Autodesk Inventor part; units mm, degrees
ref_plane "YZ Plane" through (0, 0, 0) normal (1, 0, 0) x (0, 1, 0)
ref_plane "XZ Plane" through (0, 0, 0) normal (0, 1, 0) x (-1, 0, 0)
ref_plane "XY Plane" through (0, 0, 0) normal (0, 0, 1) x (1, 0, 0)
sketch "스케치1" plane through (0, 0, 0) normal (0, 1, 0) x (-1, 0, 0)
  circle A0 centre (0, 0) radius 3.4
  dimension "d0" = 6.8
extrude "돌출1" add sketch "스케치1" along normal blind 3.8
hole "구멍1" at (0, 3.8, 0) direction (0, -1, 0) diameter 2.5 end through all
hole "구멍2" at (0, 3.8, 0) direction (0, -1, 0) diameter 4.6 depth 1.1
hole "구멍3" at (0, 0, 0) direction (0, 1, 0) diameter 4.6 depth 2.1
sketch "스케치2" plane through (0, 3.8, 0) normal (0, 1, 0) x (1, 0, 0)
  line L0 (0, 3.4) -> (0, -16)
  line L1 (-2.6, -2.1909) -> (-1.2931, -14.8337)
  arc A0 (0, 3.4) -> (-2.6, -2.1909) centre (0, 0) ccw
  arc A1 (-1.2931, -14.8337) -> (0, -16) centre (0, -14.7) ccw
  line L2 (2.6, -2.1909) -> (1.2931, -14.8337)
  arc A2 (2.6, -2.1909) -> (0, 3.4) centre (0, 0) ccw
  arc A3 (0, -16) -> (1.2931, -14.8337) centre (0, -14.7) ccw
  arc A4 (-2.6, -2.1909) -> (2.6, -2.1909) centre (0, 0) ccw
  dimension "d34" = 19.4
extrude "돌출2" add sketch "스케치2" against normal blind 1.4 contours A4 L2 A3 L0 | L0 A1 L1 A4
properties part number "SG90 SingleArm"
Design review of the part built by this model. Coordinates are the model's own, in mm. A direction names the side the tool comes from. Give positions to 0.01 mm unless a question says otherwise; leave off trailing zeros. Write each loop counter-clockwise with the first axis right and the second up, starting at its lowest first coordinate (ties: lowest second). Pieces come first, ordered by that corner, then holes. Notation, with made-up numbers: (-6, -4) - (41, -4) arc R16 ccw to (41, 27) - close; hole circle Ø3 at (-12, -35). An arc over 180 degrees is marked (long way). Return JSON: item names as keys, results as strings. Group by question number.
(1) We need section C-C, the plane y = 1.9. Give the boundary of the cut face in (x, z), then the cut area to 3 significant figures.
(2) Mouldability with a two-part tool opening along X and no side actions: class faces 4 (the cylindrical face through (1.4, 3.242, -1.825)), 5 (the flat face through (0, 3.8, 6)), 6 (the flat face through (-2, 3, 8)) as +X half, -X half, draft (parallel to the pull), parting line (faces both ways), or undercut.
(3) We need section B-B, the plane x = 1. Give the boundary of the cut face in (y, z), then the cut area to 3 significant figures.
(4) Insertion check: pin 1 (1 mm diameter, centred on y = 2.5, z = 11, fed in from +X); pin 2 (2 mm diameter, centred on x = 1, z = 11, fed in from -Y); pin 3 (4 mm diameter, centred on x = 0, z = 0, fed in from +Y); pin 4 (2 mm diameter, centred on x = 0, z = 0, fed in from +Y). Each pin has a flat end and moves straight along its axis. Give the tip position at first contact, or say it passes through.
(5) We need section A-A, the plane z = 0. Give the boundary of the cut face in (x, y).
(6) To check wall thickness, follow probe 1 along Z at (x, y) = (0, 2.55); probe 2 along Z at (x, y) = (0, 3.2); probe 3 along Y at (x, z) = (1, 6.5). State the ranges of each line that lie inside material, in increasing order.
(7) We need section D-D, the plane x = -1.5. Give the boundary of the cut face in (y, z), then the cut area to 3 significant figures.
(8) Machinability: for faces 1 (the cylindrical face through (0.44, 1.87, -3.37)), 2 (the flat face through (1, 2.7, 1)), 3 (the flat face through (2, 3, 8)), which of the approach directions +Z, -Z, +X, -X, +Y, -Y give a long, thin tool a straight path to every point of the face, cutting with its end or side? Answer none if there is none.
Reported:
{
 "1": {"outline": "circle Ø6.8 at (0, 0); hole circle Ø4.6 at (0, 0)", "area": "19.7 mm2"},
 "2": {"face 4": "undercut", "face 5": "draft", "face 6": "-X half"},
 "3": {"outline": "(0, -3.25) - (3.8, -3.25) - (3.8, -2.07) - (2.7, -2.07) - (2.7, -0.75) - (2.1, -0.75) - (2.1, -2.07) - (0, -2.07) - close; (0, 2.07) - (2.1, 2.07) - (2.1, 0.75) - (2.7, 0.75) - (2.7, 2.07) - (3.8, 2.07) - (3.8, 15.53) - (2.4, 15.53) - (2.4, 3.25) - (0, 3.25) - close", "area": "27.7 mm2"},
 "4": {"pin 1": "stops at x = 1.74", "pin 2": "stops at y = 2.4", "pin 3": "stops at y = 2.7", "pin 4": "passes through"},
 "5": {"outline": "(-3.4, 0) - (-2.3, 0) - (-2.3, 2.1) - (-1.25, 2.1) - (-1.25, 2.7) - (-2.3, 2.7) - (-2.3, 3.8) - (-3.4, 3.8) - close; (1.25, 2.1) - (2.3, 2.1) - (2.3, 0) - (3.4, 0) - (3.4, 3.8) - (2.3, 3.8) - (2.3, 2.7) - (1.25, 2.7) - close"},
 "6": {"probe 1": "z = -3.4 to -1.25, 1.25 to 16", "probe 2": "z = -3.4 to -2.3, 2.3 to 16", "probe 3": "y = 2.4 to 3.8"},
 "7": {"outline": "(0, -3.05) - (3.8, -3.05) - (3.8, -1.74) - (2.7, -1.74) - (2.7, 1.74) - (3.8, 1.74) - (3.8, 12.83) - (2.4, 12.83) - (2.4, 3.05) - (0, 3.05) - (0, 1.74) - (2.1, 1.74) - (2.1, -1.74) - (0, -1.74) - close", "area": "25.7 mm2"},
 "8": {"face 1": "-Y", "face 2": "+Y", "face 3": "+Z, +X, +Y, -Y"}
}
